Verification items for the finished model (mm, model axes). A direction names the side the tool comes from. Give positions to 0.01 mm unless a question says otherwise; leave off trailing zeros. Order: outer loops, then holes, each group sorted by start corner. A loop starts at its lowest first (then second) coordinate and runs counter-clockwise, first axis right, second up. Notation, with made-up numbers: M 71,83.5 L 105,83.5 A13 cw 105,91.5 Z; hole C 53.5,0 d11. An arc over 180 degrees is marked long. Answer as a JSON object with one key per item and string values.
```python
from build123d import *

# Parameters (mm, degrees)
F0_R     = 10.5
F1_DEPTH = 4
F2_R     = 8
F3_DEPTH = 39


with BuildPart() as f1:
    # F0 (on Top) → F1 (new body)
    with BuildSketch(Plane.XY):
        Circle(F0_R)
    extrude(amount=F1_DEPTH)

    # F2 (on Top) → F3 (join)
    with BuildSketch(Plane.XY):
        Circle(F2_R)
    extrude(amount=F3_DEPTH)

    # F4 (on Right) → F5 (revolve)
    with BuildSketch(Plane.YZ):
        with BuildLine():
            Line((4, 42), (0, 42))
            Line((0, 42), (0, 39))
            Line((0, 39), (5, 39))
            ThreePointArc((5, 39), (4.743416, 40.581139), (4, 42))
        make_face()
        with BuildLine():
            Line((0, 47), (0, 44))
            ThreePointArc((0, 44), (2.236068, 43.472136), (4, 42))
            Line((4, 42), (2, 47))
            Line((2, 47), (0, 47))
        make_face()
        with BuildLine():
            ThreePointArc((4, 42), (2.236068, 43.472136), (0, 44))
            Line((0, 44), (0, 42))
            Line((0, 42), (4, 42))
        make_face()
    revolve(axis=Axis((0, 0, 41.5), (0, 0, -1)))


solid = f1.part
```
Q1. Tool access check on faces 1 (the face through (0, 0, 0)), 2 (the face through (-1.73, -7.81, 21.26)). Record the directions out of +Z, -Z, +X, -X, +Y, -Y that give a thin tool (end or side, any length) a straight path to the whole face; none if there is none.
Resolved:
{"face 1": "-Z, +X, -X, +Y, -Y", "face 2": "+Z"}
Q2. Section check C-C on z = 43.5. Record the cut outline in (x, y), then the cut area to 3 significant figures.
Resolved:
{"outline": "C 0,0 d6.8", "area": "36.3 mm²"}
Q3. Section check A-A on y = 6.5. Record the cut outline in (x, z), then the cut area to 3 significant figures.
Resolved:
{"outline": "M -8.25,0 L 8.25,0 L 8.25,4 L 4.66,4 L 4.66,39 L -4.66,39 L -4.66,4 L -8.25,4 Z", "area": "392 mm²"}
Q4. Section check B-B on x = 7.25. Record the cut outline in (y, z), then the cut area to 3 significant figures.
Resolved:
{"outline": "M -7.6,0 L 7.6,0 L 7.6,4 L 3.38,4 L 3.38,39 L -3.38,39 L -3.38,4 L -7.6,4 Z", "area": "297 mm²"}
Q5. Section check D-D on z = 5.5. Record the cut outline in (x, y), then the cut area to 3 significant figures.
Resolved:
{"outline": "C 0,0 d16", "area": "201 mm²"}
Q6. Gauge pin test, flat ends, axial feed: pin 1 Ø1 at (x, z) = (-4, 33) entering from +Y; pin 2 Ø1 at (x, z) = (2, 11.5) entering from +Y; pin 3 Ø8 at (x, z) = (1, 8.5) entering from +Y. Record the tip position at first contact, or that the pin passes through.
Resolved:
{"pin 1": "stops at y = 7.19", "pin 2": "stops at y = 7.86", "pin 3": "stops at y = 8"}
Q7. Material ranges on L1, parallel to Z at x = -3.25, y = -8.75; L2, parallel to X at y = 0, z = 14.5; L3, parallel to Z at x = -5.25, y = -5.5, recorded low to high.
Resolved:
{"L1": "z = 0 to 4", "L2": "x = -8 to 8", "L3": "z = 0 to 39"}
